Geometry check sheet. Reference: the model listing, model coordinates, mm. Face numbers are marked on the shaded views. A direction names the side the tool comes from. Give positions to 0.01 mm unless a question says otherwise; leave off trailing zeros. Write each loop counter-clockwise with the first axis right and the second up, starting at its lowest first coordinate (ties: lowest second). Pieces come first, ordered by that corner, then holes. Notation, with made-up numbers: M 74,-10.5 L 111,-10.5 A21 ccw 111,1.5 Z; hole C 23.5,6.5 d6. An arc over 180 degrees is marked long. One line per item, written item: value. Start each with the question number.
1. Cross-section at A-A on z = 2.2. Count the separate pieces of the cut face and the enclosed holes in it, then the cut area to 3 significant figures.
2. Tool access check on the marked faces 1, 2 and 3. Record the directions out of +Z, -Z, +X, -X, +Y, -Y that give a thin tool (end or side, any length) a straight path to the whole face; none if there is none.
3. Gauge pin test, flat ends, axial feed: pin 1 (7.5 mm diameter, centred on x = 1.5, y = -0.5, fed in from +Z); pin 2 (13 mm diameter, centred on x = -4.5, y = 2, fed in from +Z). Record the tip position at first contact, or that the pin passes through.
4. Cross-section at B-B on x = 0. Record the cut outline in (y, z) (3 decimals).
5. Scan lines: line 1 (X direction, y = 4, z = 2.1); line 2 (X direction, y = 4.5, z = 1.9); line 3 (Y direction, x = 6, z = 2.2). Record each from-to range of solid material in increasing order.
6. Release check for a two-part mould opening along X. For the marked faces 4, 5 and 6 record: pulls with the +X half, pulls with the -X half, needs draft (parallel to the pull), parting line crosses it, or undercut.
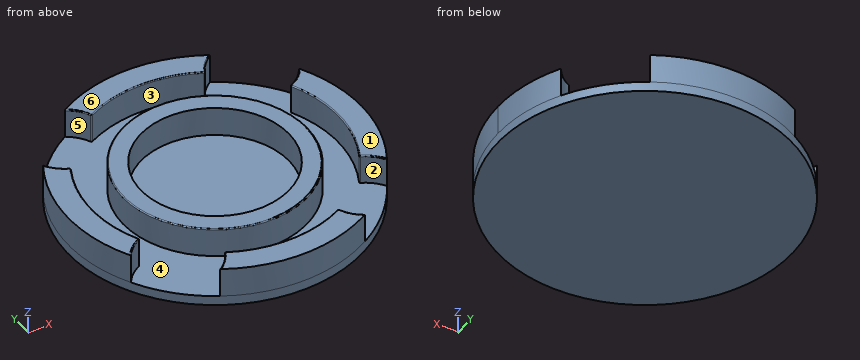
from build123d import *

# Parameters (mm, degrees)
BOSS_EXTRUDE1_DEPTH   = 3
BOSS_EXTRUDE1_2_DEPTH = 3
BOSS_EXTRUDE1_3_DEPTH = 3
BOSS_EXTRUDE1_4_DEPTH = 3
SKETCH1_R             = 9.4
SKETCH1_R_2           = 7.575
BOSS_EXTRUDE1_5_DEPTH = 3
BOSS_EXTRUDE2_START   = -1
SKETCH2_R             = 15
BOSS_EXTRUDE2_DEPTH   = 1
FILLET1_R             = 0.1
FILLET2_R             = 0.1


with BuildPart() as part:
    # Sketch1 → Boss-Extrude1 (new body)
    with BuildSketch(Plane.XY):
        with BuildLine():
            ThreePointArc((5.790318529, 11.190719876), (6.456402483, 12.241261263), (7.406868315, 13.043707363))
            ThreePointArc((7.406868315, 13.043707363), (0, 15), (-7.406868315, 13.043707363))
            ThreePointArc((-7.406868315, 13.043707363), (-6.456402483, 12.241261263), (-5.790318529, 11.190719876))
            ThreePointArc((-5.790318529, 11.190719876), (0, 12.6), (5.790318529, 11.190719876))
        make_face()
    extrude(amount=BOSS_EXTRUDE1_DEPTH)



with BuildPart() as body_2:
    # Sketch1 → Boss-Extrude1 2 (new body)
    with BuildSketch(Plane.XY):
        with BuildLine():
            ThreePointArc((13.043707363, -7.406868315), (14.502682691, -3.830430103), (15, 0))
            ThreePointArc((15, 0), (14.502682691, 3.830430103), (13.043707363, 7.406868315))
            ThreePointArc((13.043707363, 7.406868315), (12.241261263, 6.456402483), (11.190719876, 5.790318529))
            ThreePointArc((11.190719876, 5.790318529), (12.6, 0), (11.190719876, -5.790318529))
            ThreePointArc((11.190719876, -5.790318529), (12.241261263, -6.456402483), (13.043707363, -7.406868315))
        make_face()
    extrude(amount=BOSS_EXTRUDE1_2_DEPTH)


with BuildPart() as body_3:
    # Sketch1 → Boss-Extrude1 3 (new body)
    with BuildSketch(Plane.XY):
        with BuildLine():
            ThreePointArc((-7.406868315, -13.043707363), (0, -15), (7.406868315, -13.043707363))
            ThreePointArc((7.406868315, -13.043707363), (6.456402483, -12.241261263), (5.790318529, -11.190719876))
            ThreePointArc((5.790318529, -11.190719876), (0, -12.6), (-5.790318529, -11.190719876))
            ThreePointArc((-5.790318529, -11.190719876), (-6.456402483, -12.241261263), (-7.406868315, -13.043707363))
        make_face()
    extrude(amount=BOSS_EXTRUDE1_3_DEPTH)


with BuildPart() as body_4:
    # Sketch1 → Boss-Extrude1 4 (new body)
    with BuildSketch(Plane.XY):
        with BuildLine():
            ThreePointArc((-11.190719876, 5.790318529), (-12.241261263, 6.456402483), (-13.043707363, 7.406868315))
            ThreePointArc((-13.043707363, 7.406868315), (-15, 0), (-13.043707363, -7.406868315))
            ThreePointArc((-13.043707363, -7.406868315), (-12.241261263, -6.456402483), (-11.190719876, -5.790318529))
            ThreePointArc((-11.190719876, -5.790318529), (-12.6, 0), (-11.190719876, 5.790318529))
        make_face()
    extrude(amount=BOSS_EXTRUDE1_4_DEPTH)


with BuildPart() as body_5:
    # Sketch1 → Boss-Extrude1 5 (new body)
    with BuildSketch(Plane.XY):
        Circle(SKETCH1_R)
        Circle(SKETCH1_R_2, mode=Mode.SUBTRACT)
    extrude(amount=BOSS_EXTRUDE1_5_DEPTH)


with BuildPart() as part_1:
    add(part.part)

    add(body_2.part)  # Boss-Extrude2 merges body 2

    add(body_3.part)  # Boss-Extrude2 merges body 3

    add(body_4.part)  # Boss-Extrude2 merges body 4

    add(body_5.part)  # Boss-Extrude2 merges body 5
    # Sketch2 → Boss-Extrude2 (add)
    with BuildSketch(Plane.XY.offset(BOSS_EXTRUDE2_START)):
        with Locations(Location((0, 0, 0), (0, 0, 150.409926376))):
            Circle(SKETCH2_R)
    extrude(amount=BOSS_EXTRUDE2_DEPTH)

    # Fillet1
    fillet1_edges = [part_1.edges().sort_by_distance(p)[0] for p in [
        (11.190719876, 5.790318529, 1.5),
        (11.190719876, -5.790318529, 1.5),
        (5.790318529, -11.190719876, 1.5),
        (-5.790318529, -11.190719876, 1.5),
        (-11.190719876, -5.790318529, 1.5),
        (-11.190719876, 5.790318529, 1.5),
        (5.790318529, 11.190719876, 1.5),
        (-5.790318529, 11.190719876, 1.5),
    ]]
    fillet(fillet1_edges, radius=FILLET1_R)

    # Fillet2
    fillet2_edges = [part_1.edges().sort_by_distance(p)[0] for p in [
        (6.490717006, 12.280096445, 3),
        (12.280096445, -6.490717006, 3),
        (-6.490717006, -12.280096445, 3),
        (-12.280096445, 6.490717006, 3),
        (-9.4, 0, 3),
        (0, -12.6, 3),
        (6.490717006, -12.280096445, 3),
        (5.775107932, -11.232998068, 3),
        (-5.775107932, -11.232998068, 3),
        (12.6, 0, 3),
        (12.280096445, 6.490717006, 3),
        (11.232998068, 5.775107932, 3),
        (11.232998068, -5.775107932, 3),
        (0, 12.6, 3),
        (-6.490717006, 12.280096445, 3),
        (-5.775107932, 11.232998068, 3),
        (5.775107932, 11.232998068, 3),
        (-12.6, 0, 3),
        (-12.280096445, -6.490717006, 3),
        (-11.232998068, -5.775107932, 3),
        (-11.232998068, 5.775107932, 3),
    ]]
    fillet(fillet2_edges, radius=FILLET2_R - 0.0001)  # a hair under: the kernel refuses the full size


solid = part_1.part
Report:
1. separate pieces: 5
1. enclosed holes: 1
1. area: 227 mm^2
2. face 1: +Z, +X, -X, +Y, -Y
2. face 2: +Z, -Y
2. face 3: +Z
3. pin 1: stops at z = 0
3. pin 2: stops at z = 3
4. outline: M -15,-1 L 15,-1 L 15,3 L 12.7,3 A0.1 ccw 12.6,2.9 L 12.6,0 L 9.4,0 L 9.4,2.9 A0.1 ccw 9.3,3 L 7.575,3 L 7.575,0 L -7.575,0 L -7.575,3 L -9.3,3 A0.1 ccw -9.4,2.9 L -9.4,0 L -12.6,0 L -12.6,2.9 A0.1 ccw -12.7,3 L -15,3 Z
5. line 1: x = -14.46 to -11.95, -8.51 to -6.43, 6.43 to 8.51, 11.95 to 14.46
5. line 2: x = -14.31 to -11.77, -8.25 to -6.09, 6.09 to 8.25, 11.77 to 14.31
5. line 3: y = -13.75 to -11.6, -7.24 to -4.62, 4.62 to 7.24, 11.6 to 13.75
6. face 4: undercut
6. face 5: pulls with the -X half
6. face 6: needs draft
